```python
from build123d import *

# Parameters (mm, degrees)
F3_D    = 10.5
F5_D    = 22
F6_SIZE = 1


with BuildPart() as f1:
    # F0 (on Front) → F1 (revolve)
    with BuildSketch(Plane.XZ):
        Polygon((0, 85), (0, 80), (1, 80), (1, 0), (9, 0), (9, 85), align=None)
    revolve(axis=Axis((5, 0, 0), (-1, 0, 0)))

    # F3 (through all)
    with Locations(Plane.YZ.offset(9)):
        with Locations((0, 0)):
            Hole(F3_D / 2)

    # F5 (through all)
    with Locations(Plane.YZ.offset(9)):
        with Locations((0, 40), (34.6410161514, -20), (-34.6410161514, -20)):
            Hole(F5_D / 2)

    # F6
    f6_edges = [f1.edges().sort_by_distance(p)[0] for p in [
        (9, 0, -85),
        (9, -45.641016, -20),
        (9, -11, 40),
        (9, 23.641016, -20),
        (1, -45.641016, -20),
        (1, 23.641016, -20),
        (1, -11, 40),
    ]]
    chamfer(f6_edges, length=F6_SIZE)


solid = f1.part
```
Read the model definition and answer for the solid it produces. Units are mm, in the model's axes. A direction names the side the tool comes from. Coordinates: 2 decimals unless noted, no trailing zeros. Loops run counter-clockwise (first coordinate to the right, second up) from the corner with the lowest first, then second, coordinate; pieces in that order, holes last. Notation, with made-up numbers: (16.5, -17.75) - (26.5, -17.75) arc R22 ccw to (26.5, 21.25) - close; hole circle Ø7 at (-17, 81.25). An arc over 180 degrees is marked (long way). Answer in a Markdown table with one row per item.
1. Find section B-B, the plane z = 0. Write down the section's boundary in (x, y).
Conclusion:
| item | result |
|---|---|
| outline | (0, -85) - (8, -85) - (9, -84) - (9, -5.25) - (1, -5.25) - (1, -80) - (0, -80) - close; (0, 80) - (1, 80) - (1, 5.25) - (9, 5.25) - (9, 84) - (8, 85) - (0, 85) - close |
2. Find section A-A, the plane y = 0. Write down the section's boundary in (x, z), then the cut area to 3 significant figures.
Conclusion:
| item | result |
|---|---|
| outline | (0, -85) - (8, -85) - (9, -84) - (9, -5.25) - (1, -5.25) - (1, -80) - (0, -80) - close; (0, 80) - (1, 80) - (1, 52) - (2, 51) - (8, 51) - (9, 52) - (9, 84) - (8, 85) - (0, 85) - close; (1, 5.25) - (9, 5.25) - (9, 28) - (8, 29) - (2, 29) - (1, 28) - close |
| area | 1,110 mm² |
3. Find section C-C, the plane x = 5. Write down the section's boundary in (y, z), then the cut area to 3 significant figures.
Conclusion:
| item | result |
|---|---|
| outline | circle Ø170 at (0, 0); hole circle Ø22 at (-34.64, -20); hole circle Ø22 at (0, 40); hole circle Ø10.5 at (0, 0); hole circle Ø22 at (34.64, -20) |
| area | 21,500 mm² |
4. Given pin 1 (13 mm diameter, centred on y = 0, z = 40, fed in from +X); pin 2 (5 mm diameter, centred on x = 5.5, z = 44.5, fed in from -Y); pin 3 (8 mm diameter, centred on y = -30.5, z = 68, fed in from -X); pin 4 (2 mm diameter, centred on x = 7, z = 61, fed in from -Y), each flat-ended and moving along its own axis, determine where each tip first touches the part or whether it passes through.
Conclusion:
| item | result |
|---|---|
| pin 1 | passes through |
| pin 2 | stops at y = -73.9 |
| pin 3 | stops at x = 1 |
| pin 4 | stops at y = -60.21 |
5. Determine the mould class of faces 1 (the face through (3.944, -51.721, -67.453)), 2 (the face through (0, -50, 63)), 3 (the face through (0.51, -78.1, -17.34)) for opening direction Y: +Y half, -Y half, draft (parallel to the pull), parting line (faces both ways), or undercut.
Conclusion:
| item | result |
|---|---|
| face 1 | parting line |
| face 2 | draft |
| face 3 | undercut |
6. Which of the six approach directions +Z, -Z, +X, -X, +Y, -Y give full straight-line access (tool end or side, diameter ignored) to faces 4 (the face through (4.96, 24.48, -24.21)), 5 (the face through (1, 1, 17))?
Conclusion:
| item | result |
|---|---|
| face 4 | +X, -X |
| face 5 | -X |
7. Find section D-D, the plane z = -20. Count the separate pieces of the cut face and the enclosed holes in it, then the cut area to 3 significant figures.
Conclusion:
| item | result |
|---|---|
| separate pieces | 3 |
| enclosed holes | 0 |
| area | 975 mm² |
8. Straight lines are drawn through the part: line 1 (Y direction, x = 0.65, z = 0); line 2 (Y direction, x = 2.75, z = -16); line 3 (X direction, y = 42, z = 26). For each, find the intervals that lie inside material, in ascending order.
Conclusion:
| item | result |
|---|---|
| line 1 | y = -85 to -80, 80 to 85 |
| line 2 | y = -83.48 to -44.89, -24.39 to 24.39, 44.89 to 83.48 |
| line 3 | x = 1 to 9 |
